from build123d import *

# Parameters (mm, degrees)
HUB_START   = 2.2
SKETCH1_R   = 7
SKETCH1_R_2 = 3.05
HUB_DEPTH   = 4.3
ARM_START   = 6.5
SKETCH2_R   = 1.6
SKETCH2_R_2 = 0.8
ARM_DEPTH   = 2.5


with BuildPart() as part:
    # Sketch1 → Hub (new body)
    with BuildSketch(Plane.XY.offset(HUB_START)):
        with Locations(Location((0, 0, 0), (0, 0, 180))):
            Circle(SKETCH1_R)
        with Locations(Location((0, 0, 0), (0, 0, 180))):
            Circle(SKETCH1_R_2, mode=Mode.SUBTRACT)
    extrude(amount=HUB_DEPTH)

    # Sketch2 → Arm (add)
    with BuildSketch(Plane.XY.offset(ARM_START)):
        with BuildLine():
            Line((-23, 4), (23, 4))
            ThreePointArc((23, 4), (27, 0), (23, -4))
            Line((23, -4), (-23, -4))
            ThreePointArc((-23, -4), (-27, 0), (-23, 4))
        make_face()
        Circle(SKETCH2_R, mode=Mode.SUBTRACT)
        with Locations((-10, 0)):
            Circle(SKETCH2_R_2, mode=Mode.SUBTRACT)
        with Locations((-15, 0)):
            Circle(SKETCH2_R_2, mode=Mode.SUBTRACT)
        with Locations((-20, 0)):
            Circle(SKETCH2_R_2, mode=Mode.SUBTRACT)
        with Locations((10, 0)):
            Circle(SKETCH2_R_2, mode=Mode.SUBTRACT)
        with Locations((15, 0)):
            Circle(SKETCH2_R_2, mode=Mode.SUBTRACT)
        with Locations((20, 0)):
            Circle(SKETCH2_R_2, mode=Mode.SUBTRACT)
    extrude(amount=ARM_DEPTH)


solid = part.part
Source: CAD feature listing. Evaluate the final solid. Frame: model axes, mm. A direction names the side the tool comes from. Coordinates: 2 decimals unless noted, no trailing zeros. Loops run counter-clockwise (first coordinate to the right, second up) from the corner with the lowest first, then second, coordinate; pieces in that order, holes last. Notation, with made-up numbers: (62, 88.25) -> (71, 88.25) arc R19 ccw to (71, 94.25) -> close; hole circle Ø8 at (24.25, 87). An arc over 180 degrees is marked (long way). Answer in a Markdown table with one row per item. Add a question column.
Q1. Pull-direction query (X, two-part tool) for faces 1 (the face through (-27, 0, 8)), 2 (the face through (-10.59, 0.54, 7.73)), 3 (the face through (0, 4, 8)), 4 (the face through (3.047, -0.134, 4.32)); classes: pulls with the +X half, pulls with the -X half, needs draft (parallel to the pull), parting line crosses it, or undercut.
Q2. Reachability of faces 5 (the face through (-6.466, 2.681, 4.32)), 6 (the face through (0, 5, 6.5)), 7 (the face through (0, -4, 8)) from +Z, -Z, +X, -X, +Y, -Y: full face, straight path, thin tool, end or side. Return the list, or none.
Q3. Ray query, line 1 along Y through (x, z) = (0, 7.6); line 2 along Y through (x, z) = (-20, 8.3); line 3 along Z through (x, y) = (-17.5, 3.5). Return the intervals inside material, ascending.
Q4. Section A-A on x = 0. Return the cut outline in (y, z).
Q5. Section B-B on z = 7.75. Return the cut outline in (x, y).
Q6. Section C-C on y = 0. Give the number of separate pieces and of enclosed holes in the cut face, and give its area (3 significant figures).
Q7. Contact query for flat-ended pins moving along their axis: pin 1 Ø2 at (x, z) = (7.5, 8) entering from +Y; pin 2 Ø0.9 at (x, y) = (1.5, 5) entering from +Z; pin 3 Ø0.8 at (x, z) = (-3.5, 7.5) entering from -Y. Output: stop coordinate, or through.
Q8. Section D-D on x = -15. Return the cut outline in (y, z).
Computed values:
| question | item | result |
|---|---|---|
| 1 | face 1 | pulls with the -X half |
| 1 | face 2 | undercut |
| 1 | face 3 | needs draft |
| 1 | face 4 | undercut |
| 2 | face 5 | -Z |
| 2 | face 6 | +Z, +X, -X, +Y |
| 2 | face 7 | +Z, +X, -X, -Y |
| 3 | line 1 | y = -4 to -1.6, 1.6 to 4 |
| 3 | line 2 | y = -4 to -0.8, 0.8 to 4 |
| 3 | line 3 | z = 6.5 to 9 |
| 4 | outline | (-7, 2.2) -> (-3.05, 2.2) -> (-3.05, 6.5) -> (-1.6, 6.5) -> (-1.6, 9) -> (-4, 9) -> (-4, 6.5) -> (-7, 6.5) -> close; (1.6, 6.5) -> (3.05, 6.5) -> (3.05, 2.2) -> (7, 2.2) -> (7, 6.5) -> (4, 6.5) -> (4, 9) -> (1.6, 9) -> close |
| 5 | outline | (-23, -4) -> (23, -4) arc R4 ccw to (23, 4) -> (-23, 4) arc R4 ccw to start; hole circle Ø1.6 at (-20, 0); hole circle Ø1.6 at (-15, 0); hole circle Ø1.6 at (-10, 0); hole circle Ø3.2 at (0, 0); hole circle Ø1.6 at (10, 0); hole circle Ø1.6 at (15, 0); hole circle Ø1.6 at (20, 0) |
| 6 | separate pieces | 8 |
| 6 | enclosed holes | 0 |
| 6 | area | 137 mm^2 |
| 7 | pin 1 | stops at y = 4 |
| 7 | pin 2 | stops at z = 6.5 |
| 7 | pin 3 | stops at y = -4 |
| 8 | outline | (-4, 6.5) -> (-0.8, 6.5) -> (-0.8, 9) -> (-4, 9) -> close; (0.8, 6.5) -> (4, 6.5) -> (4, 9) -> (0.8, 9) -> close |
